Autodesk Inventor part; units mm, degrees
ref_plane "YZ Plane" through (0, 0, 0) normal (1, 0, 0) x (0, 1, 0)
ref_plane "XZ Plane" through (0, 0, 0) normal (0, 1, 0) x (-1, 0, 0)
ref_plane "XY Plane" through (0, 0, 0) normal (0, 0, 1) x (1, 0, 0)
sketch "Sketch1" plane through (0, 0, 0) normal (0, 0, 1) x (1, 0, 0)
  line L0 (-125, 0) -> (125, 0) construction
  line L1 (-125, -25) -> (125, -25)
  line L2 (125, 25) -> (-125, 25)
  arc A0 (-125, 25) -> (-125, -25) centre (-125, 0) ccw
  arc A1 (125, -25) -> (125, 25) centre (125, 0) ccw
  point P0 (0, 0)
  dimension "d0" = 125
  dimension "d1" = 50
extrude "Extrusion1" add sketch "Sketch1" along normal blind 78
chamfer "Chamfer1" distance 10 distance2 5 4 edges at (0, -25, 0) (150, 0, 0) (0, 25, 0) (-150, 0, 0) measured on face at (41.6667, -8.3333, 0)
chamfer "Chamfer2" distance 10 distance2 5 4 edges at (0, 25, 78) (-150, 0, 78) (0, -25, 78) (150, 0, 78) measured on face at (41.6667, -8.3333, 78)
sketch "Sketch2" plane through (0, 0, 78) normal (0, 0, 1) x (1, 0, 0)
  point P0 (0, 0)
sketch "Sketch3" plane through (0, 0, 78) normal (0, 0, 1) x (1, 0, 0)
  arc A0 (-125, 15) -> (-125, -15) centre (-125, 0) ccw
  arc A1 (125, -15) -> (125, 15) centre (125, 0) ccw
  circle A2 centre (-125, 0) radius 10
  circle A3 centre (125, 0) radius 10
  point P0 (0, 0)
  dimension "d10" = 20
  dimension "d11" = 20
extrude "Extrusion2" add sketch "Sketch3" along normal blind 5 and the other way blind 83
properties part number "Arm 2 v0.1"
Input: part model. Units: mm. Frame: model coordinates. A direction names the side the tool comes from. Coordinates: 2 decimals unless noted, no trailing zeros. Order: outer loops, then holes, each group sorted by start corner. A loop starts at its lowest first (then second) coordinate and runs counter-clockwise, first axis right, second up. Notation, with made-up numbers: M -34,37 L -14,37 A13 ccw -14,53 Z; hole C -29.75,49 d6. An arc over 180 degrees is marked long. Answer in a Markdown table with one row per item.
(1) Section query A-A, the plane x = -14. Output: boundary loops of the cut face in (y, z).
Numbers:
| item | result |
|---|---|
| outline | M -25,5 L -15,0 L 15,0 L 25,5 L 25,73 L 15,78 L -15,78 L -25,73 Z |
(2) Draft query along X for faces 4 (the cylindrical face through (149.994, 0.55, 38.524)), 5 (the flat face through (-1.75, -20.07, 2.535)), 6 (the flat face through (-2, 0, 0)). Return one class per face: pulls with the +X half, pulls with the -X half, needs draft (parallel to the pull), parting line crosses it, or undercut.
Numbers:
| item | result |
|---|---|
| face 4 | pulls with the +X half |
| face 5 | needs draft |
| face 6 | undercut |
(3) Material intervals for line 1 (Z direction, x = 74.5, y = 13.5); line 2 (X direction, y = 2.5, z = 76); line 3 (X direction, y = 2.5, z = 51), sorted ascending. Write a range as [from, to].
Numbers:
| item | result |
|---|---|
| line 1 | z = [0, 78] |
| line 2 | x = [-143.83, 143.83] |
| line 3 | x = [-149.87, 149.87] |
(4) Section query C-C, the plane z = 16. Output: boundary loops of the cut face in (x, y).
Numbers:
| item | result |
|---|---|
| outline | M -125,-25 L 125,-25 A25 ccw 125,25 L -125,25 A25 ccw Z |
(5) Section query B-B, the plane y = 0. Output: boundary loops of the cut face in (x, z).
Numbers:
| item | result |
|---|---|
| outline | M -150,5 L -140,0 L -135,0 L -135,-5 L -115,-5 L -115,0 L 115,0 L 115,-5 L 135,-5 L 135,0 L 140,0 L 150,5 L 150,73 L 140,78 L 135,78 L 135,83 L 115,83 L 115,78 L -115,78 L -115,83 L -135,83 L -135,78 L -140,78 L -150,73 Z |
(6) Access query for faces 1 (the cylindrical face through (115, 0, -2)), 2 (the flat face through (2, 25, 39)), 3 (the cylindrical face through (115, 0, 80)). Directions: +Z, -Z, +X, -X, +Y, -Y. A direction counts if a zero-diameter tool reaches every point of the face in a straight line with its end or side. Return the directions, or none.
Numbers:
| item | result |
|---|---|
| face 1 | -Z |
| face 2 | +Z, -Z, +X, -X, +Y |
| face 3 | +Z |
(7) Contact query for flat-ended pins moving along their axis: pin 1 Ø8 at (x, y) = (14.5, -13.5) entering from +Z; pin 2 Ø2 at (y, z) = (-2, 68) entering from +X; pin 3 Ø5 at (x, y) = (52.5, 12.5) entering from -Z. Output: stop coordinate, or through.
Numbers:
| item | result |
|---|---|
| pin 1 | stops at z = 78 |
| pin 2 | stops at x = 149.98 |
| pin 3 | stops at z = 0 |
